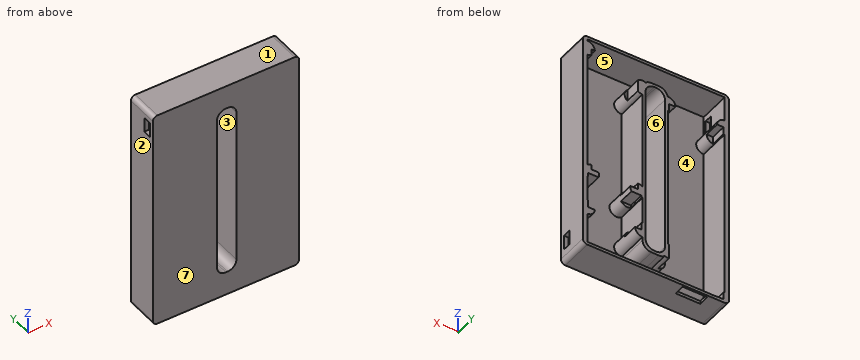
```python
from build123d import *

# Parameters (mm, degrees)
BOSS_EXTRUDE1_DEPTH = 11
SKETCH8_W           = 46
SKETCH8_H           = 73
CUT_EXTRUDE1_DEPTH  = 10.5
BOSS_EXTRUDE2_START = 10.5
SKETCH9_R           = 2.5
BOSS_EXTRUDE2_DEPTH = 10.5
SKETCH10_W          = 15.5
SKETCH10_H          = 43.25
SKETCH10_W_2        = 17.9
SKETCH10_H_2        = 12.3
SKETCH10_W_3        = 18.25
SKETCH10_H_3        = 62
CUT_EXTRUDE3_DEPTH  = 5.25
SKETCH11_W          = 5
SKETCH11_H          = 2.8
CUT_EXTRUDE4_DEPTH  = 5
SKETCH12_W          = 5
SKETCH12_H          = 2.8
CUT_EXTRUDE5_DEPTH  = 5
SKETCH14_W          = 8.25
SKETCH14_H          = 3.5
CUT_EXTRUDE6_DEPTH  = 5


with BuildPart() as part:
    # Sketch2 → Boss-Extrude1 (new body)
    with BuildSketch(Plane(origin=(0, 0, 0), x_dir=(1, 0, 0), z_dir=(0, 1, 0))):
        with BuildLine():
            Line((23, -37.5), (-23, -37.5))
            ThreePointArc((-23, -37.5), (-24.060660172, -37.060660172), (-24.5, -36))
            Line((-24.5, -36), (-24.5, 36))
            ThreePointArc((-24.5, 36), (-24.060660172, 37.060660172), (-23, 37.5))
            Line((-23, 37.5), (23, 37.5))
            ThreePointArc((23, 37.5), (24.060660172, 37.060660172), (24.5, 36))
            Line((24.5, 36), (24.5, -36))
            ThreePointArc((24.5, -36), (24.060660172, -37.060660172), (23, -37.5))
        make_face()
        with BuildLine():
            Line((0, 29.5), (0.5, 29.5))
            ThreePointArc((0.5, 29.5), (2.621320344, 28.621320344), (3.5, 26.5))
            Line((3.5, 26.5), (3.5, -26.5))
            ThreePointArc((3.5, -26.5), (2.621320344, -28.621320344), (0.5, -29.5))
            Line((0.5, -29.5), (0, -29.5))
            ThreePointArc((0, -29.5), (-2.121320344, -28.621320344), (-3, -26.5))
            Line((-3, -26.5), (-3, 26.5))
            ThreePointArc((-3, 26.5), (-2.121320344, 28.621320344), (0, 29.5))
        make_face(mode=Mode.SUBTRACT)
    extrude(amount=-BOSS_EXTRUDE1_DEPTH)

    # Sketch8 → Cut-Extrude1 (cut)
    # profile 1 of 2: a face of its own
    with BuildSketch(Plane(origin=(0, 0, 0), x_dir=(1, 0, 0), z_dir=(0, 1, 0))):
        Rectangle(SKETCH8_W, SKETCH8_H)
        with BuildLine():
            Line((-1, 30.5), (1.5, 30.5))
            ThreePointArc((1.5, 30.5), (3.621320344, 29.621320344), (4.5, 27.5))
            Line((4.5, 27.5), (4.5, -27.5))
            ThreePointArc((4.5, -27.5), (3.621320344, -29.621320344), (1.5, -30.5))
            Line((1.5, -30.5), (-1, -30.5))
            ThreePointArc((-1, -30.5), (-3.121320344, -29.621320344), (-4, -27.5))
            Line((-4, -27.5), (-4, 27.5))
            ThreePointArc((-4, 27.5), (-3.121320344, 29.621320344), (-1, 30.5))
        make_face(mode=Mode.SUBTRACT)
    # profile 2 of 2: a face of its own
    with BuildSketch(Plane(origin=(0, 0, 0), x_dir=(1, 0, 0), z_dir=(0, 1, 0))):
        with BuildLine():
            Line((0, 29.5), (0.5, 29.5))
            ThreePointArc((0.5, 29.5), (2.621320344, 28.621320344), (3.5, 26.5))
            Line((3.5, 26.5), (3.5, -26.5))
            ThreePointArc((3.5, -26.5), (2.621320344, -28.621320344), (0.5, -29.5))
            Line((0.5, -29.5), (0, -29.5))
            ThreePointArc((0, -29.5), (-2.121320344, -28.621320344), (-3, -26.5))
            Line((-3, -26.5), (-3, 26.5))
            ThreePointArc((-3, 26.5), (-2.121320344, 28.621320344), (0, 29.5))
        make_face()
    extrude(amount=-CUT_EXTRUDE1_DEPTH, mode=Mode.SUBTRACT)

    # Sketch9 → Boss-Extrude2 (add)
    with BuildSketch(Plane(origin=(0, -10.5, 0), x_dir=(1, 0, 0), z_dir=(0, 1, 0)).offset(BOSS_EXTRUDE2_START)):
        with Locations((21.58, 10.667919779)):
            Circle(SKETCH9_R)
        with Locations((6.08, 10.21529089)):
            Circle(SKETCH9_R)
        with BuildLine():
            Line((24.5, -35.456747529), (24.5, -31.456747529))
            ThreePointArc((24.5, -31.456747529), (20.5, -33.456747529), (24.5, -35.456747529))
        make_face()
        with BuildLine():
            Line((4.5, 26.342587088), (4.5, 21.342587088))
            ThreePointArc((4.5, 21.342587088), (7, 23.842587088), (4.5, 26.342587088))
        make_face()
        with BuildLine():
            Line((-4, 27.5), (-4, 25))
            ThreePointArc((-4, 25), (-6.442500859, 28.033094319), (-2.958333333, 29.772648357))
            ThreePointArc((-2.958333333, 29.772648357), (-3.727178029, 28.75), (-4, 27.5))
        make_face()
        with BuildLine():
            Line((-24.5, -27.605307327), (-24.5, -23.605307327))
            ThreePointArc((-24.5, -23.605307327), (-20.5, -25.605307327), (-24.5, -27.605307327))
        make_face()
        with BuildLine():
            Line((-20.757613835, 37.5), (-23, 37.5))
            ThreePointArc((-23, 37.5), (-24.060660172, 37.060660172), (-24.5, 36))
            Line((-24.5, 36), (-24.5, 34.394692673))
            ThreePointArc((-24.5, 34.394692673), (-21.40359225, 34.470769001), (-20.757613835, 37.5))
        make_face()
        with BuildLine():
            Line((24.5, 21.842587088), (24.5, 25.842587088))
            ThreePointArc((24.5, 25.842587088), (20.5, 23.842587088), (24.5, 21.842587088))
        make_face()
        with BuildLine():
            Line((-4, -23.105307327), (-4, -27.5))
            ThreePointArc((-4, -27.5), (-3.984574172, -27.803837144), (-3.938455326, -28.104549663))
            ThreePointArc((-3.938455326, -28.104549663), (-6.499810577, -25.636081995), (-4, -23.105307327))
        make_face()
        with BuildLine():
            Line((4.5, -25), (4.5, -27.5))
            ThreePointArc((4.5, -27.5), (4.227178029, -28.75), (3.458333333, -29.772648357))
            ThreePointArc((3.458333333, -29.772648357), (6.942500859, -28.033094319), (4.5, -25))
        make_face()
    extrude(amount=-BOSS_EXTRUDE2_DEPTH)

    # Sketch10 → Cut-Extrude3 (cut)
    with BuildSketch(Plane(origin=(0, -5.25, 0), x_dir=(1, 0, 0), z_dir=(0, 1, 0))):
        with Locations((13.83, -11.831747529)):
            Rectangle(SKETCH10_W, SKETCH10_H)
        with Locations((13.825, 17.692587088)):
            Rectangle(SKETCH10_W_2, SKETCH10_H_2)
        with Locations((-13.5, 5.394692673)):
            Rectangle(SKETCH10_W_3, SKETCH10_H_3)
    extrude(amount=CUT_EXTRUDE3_DEPTH, mode=Mode.SUBTRACT)

    # Sketch11 → Cut-Extrude4 (cut)
    with BuildSketch(Plane.ZY.offset(-23)):
        with Locations((-30.985, -8.1)):
            Rectangle(SKETCH11_W, SKETCH11_H)
    extrude(amount=-CUT_EXTRUDE4_DEPTH, mode=Mode.SUBTRACT)

    # Sketch12 → Cut-Extrude5 (cut)
    with BuildSketch(Plane(origin=(-23, 0, 0), x_dir=(0, 0, -1), z_dir=(1, 0, 0))):
        with Locations((-31.89, -8.1)):
            Rectangle(SKETCH12_W, SKETCH12_H)
    extrude(amount=-CUT_EXTRUDE5_DEPTH, mode=Mode.SUBTRACT)

    # Sketch14 → Cut-Extrude6 (cut)
    with BuildSketch(Plane.XY.offset(-36.5)):
        with Locations((-13.5, -2.4)):
            Rectangle(SKETCH14_W, SKETCH14_H)
    extrude(amount=-CUT_EXTRUDE6_DEPTH, mode=Mode.SUBTRACT)


solid = part.part
```
Could you check a few things on this model? Use its own coordinates, in mm. Face numbers are marked on the shaded views. A direction names the side the tool comes from. Give positions to 0.01 mm unless a question says otherwise; leave off trailing zeros. Loops run counter-clockwise (first coordinate to the right, second up) from the corner with the lowest first, then second, coordinate; pieces in that order, holes last. Notation, with made-up numbers: (38.5, 26) -> (49.5, 26) arc R13 ccw to (49.5, 47) -> close; hole circle Ø7 at (17.25, 75). An arc over 180 degrees is marked (long way). Put each result on its own line as item: value.
(1) Imagine slicing it at B-B on x = 14. Write out the boundary of the cut face in (y, z), plus the area to 3 significant figures.
Computed:
outline: (-11, -37.5) -> (0, -37.5) -> (0, -36.5) -> (-10.5, -36.5) -> (-10.5, 36.5) -> (0, 36.5) -> (0, 37.5) -> (-11, 37.5) -> close
area: 58.5 mm^2
(2) Thinking about a two-plate mould opening in X: for the marked faces 1, 2, 3 and 4, which applies, pulls with the +X half, pulls with the -X half, needs draft (parallel to the pull), parting line crosses it, or undercut?
Computed:
face 1: needs draft
face 2: pulls with the -X half
face 3: undercut
face 4: undercut
(3) I'm going to push flat-ended pins straight in: pin 1 Ø4 at (x, z) = (-16, 4) entering from +Y; pin 2 Ø0.7 at (x, z) = (6.5, 28.5) entering from +Y; pin 3 Ø1.1 at (y, z) = (-2.5, -37) entering from +X. Where does each tip first touch, or does it pass through?
Computed:
pin 1: y = -10.5
pin 2: y = -5.25
pin 3: x = 24.43
(4) Imagine slicing it at A-A on z = 18. Write out the boundary of the cut face in (x, y).
Computed:
outline: (-24.5, -11) -> (-3, -11) -> (-3, 0) -> (-4, 0) -> (-4, -10.5) -> (-23, -10.5) -> (-23, 0) -> (-24.5, 0) -> close; (3.5, -11) -> (24.5, -11) -> (24.5, 0) -> (23, 0) -> (23, -10.5) -> (4.5, -10.5) -> (4.5, 0) -> (3.5, 0) -> close
(5) For the marked faces 5, 6 and 7, which set-ups out of +Z, -Z, +X, -X, +Y, -Y let a thin tool reach every point of the face, with its end or its side?
Computed:
face 5: +Y
face 6: +Y, -Y
face 7: +Z, -Z, +X, -X, -Y
(6) Please list where these lines run through material, in increasing order: probe 1 along X at (y, z) = (-6.75, -17); probe 2 along Z at (x, y) = (-13.5, -6); probe 3 along Z at (x, y) = (4, -10). Write a range as [from, to].
Computed:
probe 1: [-24.5, -23], [-4, -3], [3.5, 4.5], [23, 24.5]
probe 2: [-37.5, -36.5], [36.5, 37.5]
probe 3: [-37.5, -36.5], [-29.16, 29.95], [36.5, 37.5]
(7) Imagine slicing it at C-C on y = -7.5. State how many separate pieces and enclosed holes the cut face has, plus the area to 3 significant figures.
Computed:
separate pieces: 3
enclosed holes: 1
area: 544 mm^2
